Build history of the part. All positions in model axes, mm. Face numbers are marked on the shaded views. A direction names the side the tool comes from. Give positions to 0.01 mm unless a question says otherwise; leave off trailing zeros. Write each loop counter-clockwise with the first axis right and the second up, starting at its lowest first coordinate (ties: lowest second). Pieces come first, ordered by that corner, then holes. Notation, with made-up numbers: (-30, -26.75) -> (-19, -26.75) arc R18 ccw to (-19, -8.75) -> close; hole circle Ø5 at (12, 71). An arc over 180 degrees is marked (long way). Put each result on its own line as item: value.
from build123d import *

# Parameters (mm, degrees)
BOSS_EXTRUDE1_DEPTH = 25
BOSS_EXTRUDE2_DEPTH = 25
CUT_EXTRUDE1_START  = -4.5
SKETCH3_R           = 15
CUT_EXTRUDE1_DEPTH  = 16
CHAMFER1_SIZE       = 2
FILLET2_R           = 2.5


with BuildPart() as part:
    # Sketch1 → Boss-Extrude1 (new body)
    with BuildSketch(Plane(origin=(0, 0, 0), x_dir=(0, 0, -1), z_dir=(1, 0, 0))):
        Polygon((-44.875, -95.07), (-44.875, -6.17), (-15.875, -6.17), (-15.875, 0), (15.875, 0), (15.875, -6.17), (39.625, -6.17), (39.625, -95.07), align=None)
    extrude(amount=BOSS_EXTRUDE1_DEPTH)

    # Sketch2 → Boss-Extrude2 (add)
    with BuildSketch(Plane(origin=(25, 0, 0), x_dir=(0, 0, -1), z_dir=(1, 0, 0))):
        with BuildLine():
            Line((-8.029389765, 0), (8.029389765, 0))
            ThreePointArc((8.029389765, 0), (0, 2.33), (-8.029389765, 0))
        make_face()
    extrude(amount=-BOSS_EXTRUDE2_DEPTH)

    # Sketch3 → Cut-Extrude1 (cut)
    with BuildSketch(Plane(origin=(25, 0, 0), x_dir=(0, 0, -1), z_dir=(1, 0, 0)).offset(CUT_EXTRUDE1_START)):
        with Locations((0, -12.67)):
            Circle(SKETCH3_R)
    extrude(amount=-CUT_EXTRUDE1_DEPTH, mode=Mode.SUBTRACT)

    # Chamfer1
    chamfer1_edges = [part.edges().sort_by_distance(p)[0] for p in [
        (12.5, -6.17, -39.625),
    ]]
    chamfer(chamfer1_edges, length=CHAMFER1_SIZE)

    # Fillet2
    fillet2_edges = [part.edges().sort_by_distance(p)[0] for p in [
        (12.5, 0, -8.029389765),
        (12.5, 0, 8.029389765),
    ]]
    fillet(fillet2_edges, radius=FILLET2_R)


solid = part.part
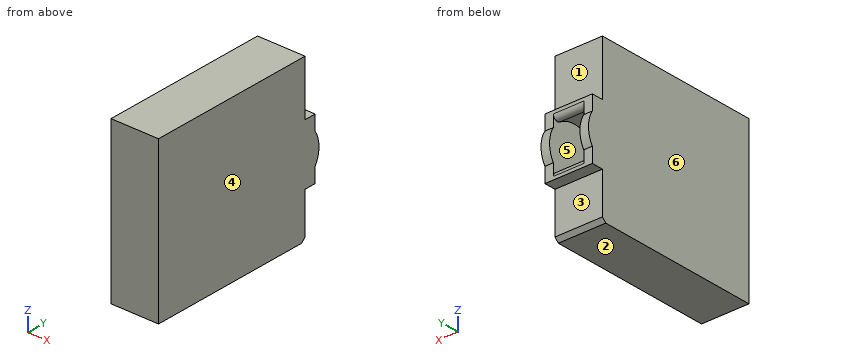
1) Wall check: L1, parallel to X at y = -8.5, z = -3; L2, parallel to Z at x = 13, y = -12.67 (3 decimals); L3, parallel to Y at x = 16.25, z = 0. Give the ranges that are in metal, low to high.
Filled sheet:
L1: 0 to 4.5, 20.5 to 25
L2: -39.625 to -15, 15 to 44.875
L3: -95.07 to -27.67
2) Tool access for the marked faces 1, 2 and 3: list every direction of +Z, -Z, +X, -X, +Y, -Y with a clear straight run to the whole face (end or side of a thin tool).
Filled sheet:
face 1: +Z, +X, -X, +Y
face 2: -Z, +X, -X, +Y, -Y
face 3: -Z, +X, -X, +Y
3) Slice it at D-D (y = -24). Write the cut outline in (x, z) (3 decimals).
Filled sheet:
outline: (0, -39.625) -> (25, -39.625) -> (25, 44.875) -> (0, 44.875) -> close; hole (4.5, -9.83) -> (20.5, -9.83) -> (20.5, 9.83) -> (4.5, 9.83) -> close
4) Slice it at A-A (y = -12.67). Write the cut outline in (x, z) (3 decimals).
Filled sheet:
outline: (0, -39.625) -> (25, -39.625) -> (25, 44.875) -> (0, 44.875) -> close; hole (4.5, -15) -> (20.5, -15) -> (20.5, 15) -> (4.5, 15) -> close
5) Slice it at B-B (x = 2.75). Write the cut outline in (y, z) (3 decimals), plus the area to 3 significant figures.
Filled sheet:
outline: (-95.07, -39.625) -> (-8.17, -39.625) -> (-6.17, -37.625) -> (-6.17, -15.875) -> (0, -15.875) -> (0, -8.029) arc R15 ccw to (0, 8.029) -> (0, 15.875) -> (-6.17, 15.875) -> (-6.17, 44.875) -> (-95.07, 44.875) -> close
area: 7,730 mm2
6) Slice it at C-C (z = 0). Write the cut outline in (x, y), plus the area to 4 significant figures.
Filled sheet:
outline: (0, -95.07) -> (25, -95.07) -> (25, 2.33) -> (20.5, 2.33) -> (20.5, -27.67) -> (4.5, -27.67) -> (4.5, 2.33) -> (0, 2.33) -> close
area: 1,955 mm2
7) Pin check, flat tips, straight feed: pin 1 (4 mm diameter, centred on x = 11, z = -13, fed in from +Y); pin 2 (1.9 mm diameter, centred on x = 11, y = -1.5, fed in from -Z) (3 decimals); pin 3 (1.9 mm diameter, centred on x = 9, y = -2, fed in from +Z) (3 decimals). Stop position of each tip, or through.
Filled sheet:
pin 1: y = 0
pin 2: z = -15.875
pin 3: z = 15.875
8) Pull direction X, two halves, no side cores. Call the marked faces 4, 5 and 6: released by +X, released by -X, zero draft, split by the parting line, or undercut.
Filled sheet:
face 4: released by +X
face 5: undercut
face 6: released by -X
